CAD build for the part. Positions are in the model's coordinates, mm. A direction names the side the tool comes from. Round coordinates to 2 decimals unless told otherwise and drop trailing zeros. Order: outer loops, then holes, each group sorted by start corner. A loop starts at its lowest first (then second) coordinate and runs counter-clockwise, first axis right, second up. Notation, with made-up numbers: (-10.75, 11.25) - (44.25, 11.25) arc R24 ccw to (44.25, 26.25) - close; hole circle Ø4 at (-17, -35.5). An arc over 180 degrees is marked (long way). Write item = value, one per line.
from build123d import *

# Parameters (mm, degrees)
ESBO_O1_W                    = 80
ESBO_O1_H                    = 40
RESSALTO_EXTRUS_O1_DEPTH     = 80
ESBO_O2_W                    = 20
ESBO_O2_H                    = 40
CORTE_EXTRUS_O1_DEPTH        = 80
FILETE1_RADIUS               = 20
FILETE1_LENGTH               = 40
FURO_DE_DI_METRO_20_0_20_1_D = 20
CHANFRO1_SIZE                = 1
CORTE_EXTRUS_O2_DEPTH        = 80
CORTE_EXTRUS_O3_DEPTH        = 80
FILETE2_R                    = 2
FILETE3_R                    = 5


with BuildPart() as part:
    # Esboço1 → Ressalto-extrusão1 (new body)
    with BuildSketch(Plane(origin=(0, 0, 0), x_dir=(1, 0, 0), z_dir=(0, 1, 0))):
        Rectangle(ESBO_O1_W, ESBO_O1_H)
    extrude(amount=RESSALTO_EXTRUS_O1_DEPTH)

    # Esboço2 → Corte-extrusão1 (cut)
    with BuildSketch(Plane.XY.offset(20)):
        with Locations((-30, 60)):
            Rectangle(ESBO_O2_W, ESBO_O2_H)
        with Locations((30, 60)):
            Rectangle(ESBO_O2_W, ESBO_O2_H)
    extrude(amount=-CORTE_EXTRUS_O1_DEPTH, mode=Mode.SUBTRACT)

    # Filete1: full round fillet: the end face becomes a half cylinder, R = half its width
    filete1_face = Plane((0, 80, 0), x_dir=(0, 0, -1), z_dir=(0, 1, 0))  # on the end face: x along it, z out of the body
    filete1_slab = filete1_face.offset(-FILETE1_RADIUS / 2) * Box(FILETE1_LENGTH, 2 * FILETE1_RADIUS, FILETE1_RADIUS, mode=Mode.PRIVATE)  # the body's end, R deep
    filete1_round = Plane((0, 60, 0), x_dir=(0, 1, 0), z_dir=(0, 0, -1)) * Cylinder(FILETE1_RADIUS, FILETE1_LENGTH, mode=Mode.PRIVATE)  # its axis R under the face
    add(filete1_slab - filete1_round, mode=Mode.SUBTRACT)

    # Furo de diâmetro Ø20.0 (20)1 (through all)
    with Locations(Plane.XY.offset(20)):
        with Locations((0, 60)):
            Hole(FURO_DE_DI_METRO_20_0_20_1_D / 2)

    # Chanfro1
    chanfro1_edges = [part.edges().sort_by_distance(p)[0] for p in [
        (10, 60, 20),
        (10, 60, -20),
    ]]
    chamfer(chanfro1_edges, length=CHANFRO1_SIZE)

    # Esboço5 → Corte-extrusão2 (cut)
    with BuildSketch(Plane(origin=(0, 40, 0), x_dir=(1, 0, 0), z_dir=(0, 1, 0))):
        Polygon((40, 15), (35, 15), (27, 0), (35, -15), (40, -15), align=None)
    corte_extrus_o2 = extrude(amount=-CORTE_EXTRUS_O2_DEPTH, mode=Mode.SUBTRACT)

    # Espelhar1: Corte-extrusão2 across plane
    add(corte_extrus_o2.mirror(Plane(origin=(0, 0, 0), x_dir=(0, 0, 1), z_dir=(1, 0, 0))), mode=Mode.SUBTRACT)

    # Esboço6 → Corte-extrusão3 (cut)
    with BuildSketch(Plane.XY.offset(20)):
        Polygon((-13, 0), (-13, 15), (-20, 15), (-20, 30), (20, 30), (20, 15), (13, 15), (13, 0), align=None)
    extrude(amount=-CORTE_EXTRUS_O3_DEPTH, mode=Mode.SUBTRACT)

    # Filete2
    filete2_edges = [part.edges().sort_by_distance(p)[0] for p in [
        (-20, 15, 0),
        (-20, 30, 0),
        (20, 30, 0),
        (20, 15, 0),
    ]]
    fillet(filete2_edges, radius=FILETE2_R)

    # Filete3
    filete3_edges = [part.edges().sort_by_distance(p)[0] for p in [
        (-20, 40, 0),
        (20, 40, 0),
    ]]
    fillet(filete3_edges, radius=FILETE3_R)


solid = part.part
(1) Probe line 1 along Y through (x, z) = (0, -3.5); line 2 along Z through (x, y) = (37, 29); line 3 along Y through (x, z) = (-28, 16.5). List the from-to ranges inside material, lowest first.
Solved:
line_1 = 30 to 50, 70 to 80
line_2 = -20 to -15, 15 to 20
line_3 = 0 to 40
(2) Tool access for faces 4 (the flat face through (29, 40, 5)), 5 (the flat face through (13, 8, 0)), 6 (the flat face through (31.056, 20.28, -7.605)): list every direction of +Z, -Z, +X, -X, +Y, -Y with a clear straight run to the whole face (end or side of a thin tool).
Solved:
face_4 = +Z, -Z, +X, +Y
face_5 = +Z, -Z, -Y
face_6 = +X, +Y, -Y
(3) Band-saw the part on C-C on y = 46. List the corners of the cut face in (x, z), plus the area to 3 significant figures.
Solved:
outline = (-20, -20) - (20, -20) - (20, 20) - (-20, 20) - close
area = 1,600 mm²
(4) Band-saw the part on B-B on z = 9. List the corners of the cut face in (x, y).
Solved:
outline = (-31.8, 0) - (-13, 0) - (-13, 15) - (-18, 15) arc R2 cw to (-20, 17) - (-20, 28) arc R2 cw to (-18, 30) - (18, 30) arc R2 cw to (20, 28) - (20, 17) arc R2 cw to (18, 15) - (13, 15) - (13, 0) - (31.8, 0) - (31.8, 40) - (25, 40) arc R5 cw to (20, 45) - (20, 60) arc R20 ccw to (-20, 60) - (-20, 45) arc R5 cw to (-25, 40) - (-31.8, 40) - close; hole circle Ø20 at (0, 60)
(5) Drop flat-ended pins along their axis: pin 1 (5.5 mm diameter, centred on y = 23.5, z = -7, fed in from +X); pin 2 (12 mm diameter, centred on y = 54.5, z = 1.5, fed in from +X); pin 3 (4.5 mm diameter, centred on y = 54, z = -3.5, fed in from -X); pin 4 (16 mm diameter, centred on x = 0, y = 60, fed in from -Z). Give the stop position or say it passes through.
Solved:
pin_1 = 32.2
pin_2 = 20
pin_3 = -20
pin_4 = through
(6) Band-saw the part on D-D on z = -7.5. List the corners of the cut face in (x, y), plus the area to 3 significant figures.
Solved:
outline = (-31, 0) - (-13, 0) - (-13, 15) - (-18, 15) arc R2 cw to (-20, 17) - (-20, 28) arc R2 cw to (-18, 30) - (18, 30) arc R2 cw to (20, 28) - (20, 17) arc R2 cw to (18, 15) - (13, 15) - (13, 0) - (31, 0) - (31, 40) - (25, 40) arc R5 cw to (20, 45) - (20, 60) arc R20 ccw to (-20, 60) - (-20, 45) arc R5 cw to (-25, 40) - (-31, 40) - close; hole circle Ø20 at (0, 60)
area = 2,620 mm²
(7) Band-saw the part on A-A on x = 0. List the corners of the cut face in (y, z), plus the area to 3 significant figures.
Solved:
outline = (30, -20) - (49, -20) - (50, -19) - (50, 19) - (49, 20) - (30, 20) - close; (70, -19) - (71, -20) - (80, -20) - (80, 20) - (71, 20) - (70, 19) - close
area = 1,200 mm²
(8) Pull direction Z, two halves, no side cores. Call faces 1 (the flat face through (-37, 20, 15)), 2 (the flat face through (-1, 31, 20)), 3 (the cylindrical face through (-19.43, 29.4, -0.28)): released by +Z, released by -Z, zero draft, split by the parting line, or undercut.
Solved:
face_1 = undercut
face_2 = released by +Z
face_3 = zero draft
